Autodesk Inventor part; units mm, degrees
ref_plane "YZ Plane" through (0, 0, 0) normal (1, 0, 0) x (0, 1, 0)
ref_plane "XZ Plane" through (0, 0, 0) normal (0, 1, 0) x (-1, 0, 0)
ref_plane "XY Plane" through (0, 0, 0) normal (0, 0, 1) x (1, 0, 0)
sketch "Esquisse1" plane through (0, 0, 0) normal (0, 1, 0) x (-1, 0, 0)
  line L0 (-42, -42) -> (42, -42)
  line L1 (42, -42) -> (42, 42)
  line L2 (42, 42) -> (-42, 42)
  line L3 (-42, 42) -> (-42, -42)
  line L4 (-42, -42) -> (42, 42) construction
  line L5 (42, -42) -> (-42, 42) construction
  point P0 (0, 0)
  dimension "d0" = 84
  dimension "d1" = 84
extrude "Extrusion1" add sketch "Esquisse1" along normal blind 2
sketch "Esquisse2" plane through (0, 2, 0) normal (0, 1, 0) x (1, 0, 0)
  line L0 (40, 40) -> (-40, 40)
  line L1 (-40, 40) -> (-40, -40)
  line L2 (-40, -40) -> (40, -40)
  line L3 (40, 40) -> (-40, -40) construction
  line L4 (-40, 40) -> (40, -40) construction
  line L5 (40, -40) -> (42, -40)
  line L6 (42, -42) -> (42, 42)
  line L7 (40, 40) -> (42, 40)
  line L8 (-42, -42) -> (42, -42)
  line L9 (-42, 42) -> (-42, -42)
  line L10 (42, 42) -> (-42, 42)
  point P0 (0, 0)
  dimension "d4" = 2
  dimension "d5" = 2
extrude "Extrusion2" add sketch "Esquisse2" along normal blind 31 contours L0 L1 L2 L5 L6 L8 L9 L10 L7
sketch "Esquisse3" plane through (0, 33, 0) normal (0, 1, 0) x (1, 0, 0)
  line L0 (42, 40) -> (42, 42)
  line L1 (-42, -42) -> (42, -42)
  line L2 (42, -42) -> (42, 42)
  line L3 (42, 42) -> (-42, 42)
  line L4 (-42, 42) -> (-42, -42)
  point P0 (0, 0)
extrude "Extrusion3" add sketch "Esquisse3" along normal blind 2
fillet "Congé1" radius 2 4 edges at (0, 35, 42) (0, 35, -42) (0, 0, 42) (0, 0, -42)
sketch "Esquisse5" plane through (-42, 0, -40) normal (-1, 0, 0) x (0, 0, 1)
  line L0 (40, 0) -> (40, 35.2291) construction
  circle A0 centre (40, 17.6146) radius 5
  dimension "d12" = 10
extrude "Extrusion4" cut sketch "Esquisse5" against normal blind 31
properties part number "BatterieHolder_Impression 3D"
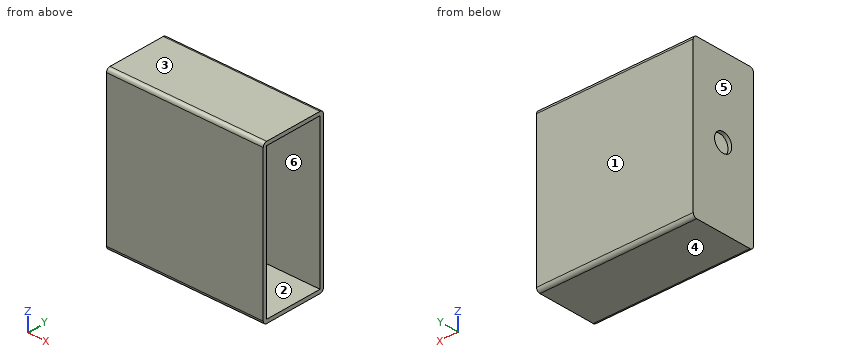
Can you work these out from the model? Positions are in its coordinate system, mm. Face numbers are marked on the shaded views. A direction names the side the tool comes from. Coordinates: 2 decimals unless noted, no trailing zeros. Write each loop counter-clockwise with the first axis right and the second up, starting at its lowest first coordinate (ties: lowest second). Pieces come first, ordered by that corner, then holes.
Q1. Imagine slicing it at A-A, the plane z = 0. List the corners of the cut face in (x, y) for me, plus the area to 3 significant figures.
Results found:
outline: (-42, 0) - (42, 0) - (42, 2) - (-40, 2) - (-40, 12.61) - (-42, 12.61) - close; (-42, 22.61) - (-40, 22.61) - (-40, 33) - (42, 33) - (42, 35) - (-42, 35) - close
area: 378 mm2
Q2. Please list where these lines run through material, in increasing order: L1, parallel to Z at x = -22.5, y = 21.5; L2, parallel to Y at x = 9.5, z = 9; L3, parallel to Y at x = -41, z = 0.
Results found:
L1: z = -42 to -40, 40 to 42
L2: y = 0 to 2, 33 to 35
L3: y = 0 to 12.61, 22.61 to 35
Q3. Imagine slicing it at D-D, the plane z = -28. List the corners of the cut face in (x, y) for me, plus the area to 3 significant figures.
Results found:
outline: (-42, 0) - (42, 0) - (42, 2) - (-40, 2) - (-40, 33) - (42, 33) - (42, 35) - (-42, 35) - close
area: 398 mm2
Q4. Which directions (+Z, -Z, +X, -X, +Y, -Y) give clear straight access to the entire face, cutting with the end or side of a thin tool? Please do the marked faces 5 and 6.
Results found:
face 5: +Z, -Z, -X, +Y, -Y
face 6: +X
Q5. Imagine slicing it at C-C, the plane y = 31. List the corners of the cut face in (x, z) for me.
Results found:
outline: (-42, -42) - (42, -42) - (42, -40) - (-40, -40) - (-40, 40) - (42, 40) - (42, 42) - (-42, 42) - close
Q6. If we mould it in two halves opening along Z, with no side actions, what happens to the marked faces 1, 2, 3 and 4? For each: +Z half, -Z half, draft (parallel to the pull), parting line (faces both ways), or undercut.
Results found:
face 1: draft
face 2: undercut
face 3: +Z half
face 4: -Z half
Q7. Imagine slicing it at B-B, the plane x = -16.5. List the corners of the cut face in (y, z) for me, plus the area to 3 significant figures.
Results found:
outline: (0, -40) arc R2 ccw to (2, -42) - (33, -42) arc R2 ccw to (35, -40) - (35, 40) arc R2 ccw to (33, 42) - (2, 42) arc R2 ccw to (0, 40) - close; hole (2, -40) - (33, -40) - (33, 40) - (2, 40) - close
area: 457 mm2
Q8. For P1, Ø15.5, axis at y = 13, z = 10, coming from the +X side, with a flat end and sliding along its axis, tell me the tip position at first contact or that it passes through.
Results found:
P1: stops at x = -40
